Here's how the part is built. I have some questions about the finished solid (model axes, mm). A direction names the side the tool comes from. Coordinates: 2 decimals unless noted, no trailing zeros. Loops run counter-clockwise (first coordinate to the right, second up) from the corner with the lowest first, then second, coordinate; pieces in that order, holes last. Notation, with made-up numbers: M -25,-30.75 L 18,-30.75 A30 cw 18,-8.75 Z; hole C -40,-35 d7. An arc over 180 degrees is marked long. Use one line per item in the form item = value. Start each with the question number.
(1) Thinking about a two-plate mould opening in X: for faces 5 (the cylindrical face through (0, 0, 29)), 6 (the flat face through (-8.5, 0, 3)), 7 (the flat face through (0, -6.5, 3)), which applies, +X half, -X half, draft (parallel to the pull), parting line (faces both ways), or undercut?
(2) Imagine slicing it at C-C, the plane x = -21. Please give me the cut outline in (y, z).
(3) On a 3-axis mill with a long thin cutter (end or side, diameter ignored), from which of +Z, -Z, +X, -X, +Y, -Y can I reach the whole of each face in a straight line? I mean faces 1 (the cylindrical face through (3.36, -5.01, 20.77)), 2 (the flat face through (-5, 5, 11)), 3 (the flat face through (0, 6.5, 3)), 4 (the flat face through (24, 0, 5)). Say none if no direction works.
(4) Please list where these lines run through material, in increasing order: L1, parallel to Y at x = -21, z = 1.35; L2, parallel to Z at x = -19, y = 4.75; L3, parallel to Y at x = -11, z = 14.5.
(5) Will these pins go through, and if not, where does the flat tip stop? P1, Ø3, axis at x = 21, y = 0, coming from the -Z side; P2, Ø6, axis at x = -15, z = 9.5, coming from the +Y side; P3, Ø4, axis at x = 22, y = 2, coming from the +Z side; P4, Ø3, axis at y = 3, z = 9.5, coming from the +X side.
```python
from build123d import *

# Parameters (mm, degrees)
F0_R          = 4
F1_DEPTH      = 6.5
F1_DEPTH_BACK = 6.5
F2_R          = 2.5
F3_DEPTH      = 25
F4_R          = 1
F5_R          = 11.25
F5_R_2        = 6.25
F6_DEPTH      = 2
F7_R          = 11.25
F7_R_2        = 6.25
F8_DEPTH      = 1.5
F9_R          = 1


with BuildPart() as f1:
    # F0 (on Front) → F1 (new body, two sides)
    with BuildSketch(Plane.XZ) as f1_sk:
        with BuildLine():
            Line((-27.5, 5), (-27.5, 0))
            Line((-27.5, 0), (-8.5, 0))
            Line((-8.5, 0), (-8.5, 5))
            Line((-8.5, 5), (-8.5, 5.011912))
            ThreePointArc((-8.5, 5.011912), (-8.492643, 5.005953), (-8.485281, 5))
            ThreePointArc((-8.485281, 5), (0, 2), (8.485281, 5))
            ThreePointArc((8.485281, 5), (8.492643, 5.005953), (8.5, 5.011912))
            Line((8.5, 5.011912), (8.5, 5))
            Line((8.5, 5), (8.5, 0))
            Line((8.5, 0), (27.5, 0))
            Line((27.5, 0), (27.5, 5))
            Line((27.5, 5), (13.5, 5))
            Line((13.5, 5), (13.5, 15.5))
            ThreePointArc((13.5, 15.5), (0, 29), (-13.5, 15.5))
            Line((-13.5, 15.5), (-13.5, 5))
            Line((-13.5, 5), (-27.5, 5))
        make_face()
        with Locations((0, 15.5)):
            Circle(F0_R, mode=Mode.SUBTRACT)
        with BuildLine():
            Line((-8.5, 5.011912), (-8.5, 5))
            Line((-8.5, 5), (-8.485281, 5))
            ThreePointArc((-8.485281, 5), (-8.492643, 5.005953), (-8.5, 5.011912))
        make_face()
        with BuildLine():
            ThreePointArc((8.5, 5.011912), (8.492643, 5.005953), (8.485281, 5))
            Line((8.485281, 5), (8.5, 5))
            Line((8.5, 5), (8.5, 5.011912))
        make_face()
    extrude(amount=F1_DEPTH)
    extrude(f1_sk.sketch, amount=-F1_DEPTH_BACK)

    # F2 (on face) → F3 (cut)
    with BuildSketch(Plane.XY.offset(5)):
        with Locations((-21, 0)):
            Circle(F2_R)
        with Locations((21, 0)):
            Circle(F2_R)
    extrude(amount=-F3_DEPTH, mode=Mode.SUBTRACT)

    # F4
    f4_edges = [f1.edges().sort_by_distance(p)[0] for p in [
        (-27.5, -6.5, 2.5),
        (-27.5, 6.5, 2.5),
        (27.5, -6.5, 2.5),
        (27.5, 6.5, 2.5),
        (13.5, 0, 5),
        (8.5, 0, 0),
        (-8.5, 0, 0),
        (-13.5, 0, 5),
    ]]
    fillet(f4_edges, radius=F4_R)

    # F5 (on face) → F6 (cut)
    with BuildSketch(Plane.XZ.offset(6.5)):
        with Locations((0, 15.5)):
            Circle(F5_R)
        with Locations((0, 15.5)):
            Circle(F5_R_2, mode=Mode.SUBTRACT)
    extrude(amount=-F6_DEPTH, mode=Mode.SUBTRACT)

    # F7 (on face) → F8 (cut)
    with BuildSketch(Plane(origin=(0, 6.5, 0), x_dir=(-1, 0, 0), z_dir=(0, 1, 0))):
        with Locations((0, 15.5)):
            Circle(F7_R)
        with Locations((0, 15.5)):
            Circle(F7_R_2, mode=Mode.SUBTRACT)
    extrude(amount=-F8_DEPTH, mode=Mode.SUBTRACT)

    # F9
    f9_edges = [f1.edges().sort_by_distance(p)[0] for p in [
        (11.25, 6.5, 15.5),
        (6.25, 6.5, 15.5),
        (-11.25, -6.5, 15.5),
        (-6.25, -6.5, 15.5),
    ]]
    fillet(f9_edges, radius=F9_R)


solid = f1.part
```
Answer:
q1.face_5 = parting line
q1.face_6 = undercut
q1.face_7 = draft
q2.outline = M -6.5,0 L -2.5,0 L -2.5,5 L -6.5,5 Z; M 2.5,0 L 6.5,0 L 6.5,5 L 2.5,5 Z
q3.face_1 = -Y
q3.face_2 = +Y
q3.face_3 = +Z, -Z, +X, -X, +Y
q3.face_4 = +Z, +X, +Y, -Y
q4.L1 = -6.5 to -2.5, 2.5 to 6.5
q4.L2 = 0 to 5
q4.L3 = -4.5 to 5
q5.P1 = through
q5.P2 = 6.5
q5.P3 = 5
q5.P4 = 13.5
